Check sheet for the modelled part. Datum: model origin and axes. Units: mm. Round coordinates to 2 decimals unless told otherwise and drop trailing zeros. Loops run counter-clockwise (first coordinate to the right, second up) from the corner with the lowest first, then second, coordinate; pieces in that order, holes last. Notation, with made-up numbers: (27.25, 87) -> (44.25, 87) arc R21 ccw to (44.25, 105) -> close; hole circle Ø2 at (5, 87.25). An arc over 180 degrees is marked (long way). One line per question, with ' | ' between items.
```python
from build123d import *

# Parameters (mm, degrees)
PAD_DEPTH       = 4
PAD001_DEPTH    = 38
PAD002_DEPTH    = 12
SKETCH009_R     = 1.4
POCKET001_DEPTH = 8


with BuildPart() as part:
    # Sketch → Pad (new body)
    with BuildSketch(Plane.XY):
        with BuildLine():
            Line((-106, 65), (106, 65))
            ThreePointArc((110, 61), (108.828427, 63.828427), (106, 65))
            Line((110, 61), (110, -61))
            ThreePointArc((106, -65), (108.828427, -63.828427), (110, -61))
            Line((106, -65), (-106, -65))
            ThreePointArc((-110, -61), (-108.828427, -63.828427), (-106, -65))
            Line((-110, -61), (-110, 61))
            ThreePointArc((-106, 65), (-108.828427, 63.828427), (-110, 61))
        make_face()
        with BuildLine():
            ThreePointArc((-97, -9), (-99.828427, -10.171573), (-101, -13))
            Line((-101, -53), (-101, -13))
            ThreePointArc((-101, -53), (-99.828427, -55.828427), (-97, -57))
            Line((97, -57), (-97, -57))
            ThreePointArc((97, -57), (99.828427, -55.828427), (101, -53))
            Line((101, -13), (101, -53))
            ThreePointArc((101, -13), (99.828427, -10.171573), (97, -9))
            Line((-97, -9), (97, -9))
        make_face(mode=Mode.SUBTRACT)
        with BuildLine():
            ThreePointArc((-97, 56), (-99.828427, 54.828427), (-101, 52))
            Line((-101, 13), (-101, 52))
            ThreePointArc((-101, 13), (-99.828427, 10.171573), (-97, 9))
            Line((97, 9), (-97, 9))
            ThreePointArc((97, 9), (99.828427, 10.171573), (101, 13))
            Line((101, 52), (101, 13))
            ThreePointArc((101, 52), (99.828427, 54.828427), (97, 56))
            Line((-97, 56), (97, 56))
        make_face(mode=Mode.SUBTRACT)
    extrude(amount=PAD_DEPTH)

    # Sketch006 (on Face26 of Pad) → Pad001 (join)
    with BuildSketch(Plane.XY.offset(4)):
        with BuildLine():
            ThreePointArc((105, 65), (104.292893, 64.707107), (104, 64))
            Line((104, -8), (104, 64))
            ThreePointArc((104, -8), (104.292893, -8.707107), (105, -9))
            Line((110, -9), (105, -9))
            Line((110, 61), (110, -9))
            ThreePointArc((110, 61), (108.828427, 63.828427), (106, 65))
            Line((105, 65), (106, 65))
        make_face()
    extrude(amount=PAD001_DEPTH)

    # Sketch008 → Pad002 (join)
    with BuildSketch(Plane.XY.offset(4)):
        with BuildLine():
            ThreePointArc((-109, 54.5), (-109.707107, 54.207107), (-110, 53.5))
            Line((-110, 41.5), (-110, 53.5))
            ThreePointArc((-110, 41.5), (-109.707107, 40.792893), (-109, 40.5))
            Line((-105, 40.5), (-109, 40.5))
            ThreePointArc((-105, 40.5), (-104.292893, 40.792893), (-104, 41.5))
            Line((-104, 53.5), (-104, 41.5))
            ThreePointArc((-104, 53.5), (-104.292893, 54.207107), (-105, 54.5))
            Line((-109, 54.5), (-105, 54.5))
        make_face()
        with BuildLine():
            ThreePointArc((-109, -40.5), (-109.707107, -40.792893), (-110, -41.5))
            Line((-110, -53.5), (-110, -41.5))
            ThreePointArc((-110, -53.5), (-109.707107, -54.207107), (-109, -54.5))
            Line((-105, -54.5), (-109, -54.5))
            ThreePointArc((-105, -54.5), (-104.292893, -54.207107), (-104, -53.5))
            Line((-104, -41.5), (-104, -53.5))
            ThreePointArc((-104, -41.5), (-104.292893, -40.792893), (-105, -40.5))
            Line((-109, -40.5), (-105, -40.5))
        make_face()
    extrude(amount=PAD002_DEPTH)

    # Sketch009 (on Face7 of Pad002) → Pocket001 (cut)
    with BuildSketch(Plane(origin=(-110, 0, 0), x_dir=(0, -1, 0), z_dir=(-1, 0, 0))):
        with Locations((2, 9)):
            Circle(SKETCH009_R)
        with Locations((97, 9)):
            Circle(SKETCH009_R)
    extrude(amount=-POCKET001_DEPTH, mode=Mode.SUBTRACT)


solid = part.part
```
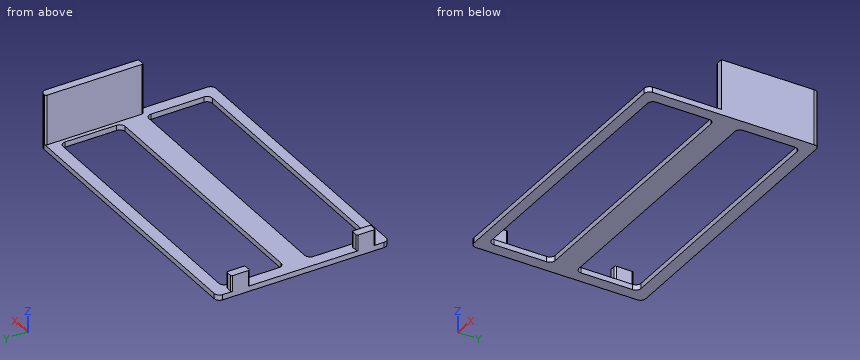
(1) Sectioned sample at B-B, the plane y = 49.5. Record the cut outline in (x, z), and give its area (3 significant figures).
Answer:
outline: (-110, 0) -> (-101, 0) -> (-101, 4) -> (-104, 4) -> (-104, 16) -> (-110, 16) -> close; (101, 0) -> (110, 0) -> (110, 42) -> (104, 42) -> (104, 4) -> (101, 4) -> close | area: 372 mm2
(2) Go/stop test with flat-tipped pins: pin 1 (5 mm diameter, centred on x = -106, y = 45, fed in from +Z); pin 2 (3.5 mm diameter, centred on y = -45.5, z = 9, fed in from +X); pin 3 (1.2 mm diameter, centred on x = -106.5, z = 12.5, fed in from +Y). Record where each tip stops, or that it passes through.
Answer:
pin 1: stops at z = 16 | pin 2: stops at x = -104 | pin 3: stops at y = 54.5
(3) Sectioned sample at C-C, the plane z = 35.5. Record the cut outline in (x, y).
Answer:
outline: (104, -8) arc R1 ccw to (105, -9) -> (110, -9) -> (110, 61) arc R4 ccw to (106, 65) -> (105, 65) arc R1 ccw to (104, 64) -> close
(4) Sectioned sample at A-A, the plane x = -77.5. Record the cut outline in (y, z).
Answer:
outline: (-65, 0) -> (-57, 0) -> (-57, 4) -> (-65, 4) -> close; (-9, 0) -> (9, 0) -> (9, 4) -> (-9, 4) -> close; (56, 0) -> (65, 0) -> (65, 4) -> (56, 4) -> close
(5) Scan lines: probe 1 along Y at (x, z) = (-23.5, 2.5); probe 2 along Z at (x, y) = (24, -0.5); probe 3 along X at (y, z) = (18, 31). Record each from-to range of solid material in increasing order.
Answer:
probe 1: y = -65 to -57, -9 to 9, 56 to 65 | probe 2: z = 0 to 4 | probe 3: x = 104 to 110
(6) Sectioned sample at D-D, the plane y = -2. Record the cut outline in (x, z), and give its area (3 significant figures).
Answer:
outline: (-110, 0) -> (110, 0) -> (110, 42) -> (104, 42) -> (104, 4) -> (-110, 4) -> close | area: 1,110 mm2
